Geometry: final body of the model. Coordinates: model frame, mm. A direction names the side the tool comes from. Round coordinates to 2 decimals unless told otherwise and drop trailing zeros. Loops run counter-clockwise (first coordinate to the right, second up) from the corner with the lowest first, then second, coordinate; pieces in that order, holes last. Notation, with made-up numbers: (22, 35) -> (65, 35) arc R32 ccw to (65, 67) -> close; hole circle Ø3 at (43, -6). An arc over 180 degrees is marked (long way). Answer in a Markdown table with one row per item.
```python
from build123d import *

# Parameters (mm, degrees)
AXIAL_START       = 9.7
SKETCH2_R         = 1.65
AXIAL_HOLES_DEPTH = 4


with BuildPart() as part:
    # Axial profile (mm) → Full revolution (revolve)
    with BuildSketch(Plane.XY, mode=Mode.PRIVATE) as full_revolution_sk:
        Polygon((-126, 52), (9.7, 52), (9.7, 32), (13.7, 32), (13.7, 55), (-126, 55), align=None)
    revolve(full_revolution_sk.sketch.rotate(Axis((-110, 0, 0), (1, 0, 0)), 90), axis=Axis((-110, 0, 0), (1, 0, 0)))

    # Sketch2 → Axial holes (cut)
    with BuildSketch(Plane(origin=(0, 0, 0), x_dir=(0, 0, -1), z_dir=(1, 0, 0)).offset(AXIAL_START)):
        with Locations((-34.648232278, 34.648232278)):
            Circle(SKETCH2_R)
        with Locations((-34.648232278, -34.648232278)):
            Circle(SKETCH2_R)
        with Locations((34.648232278, -34.648232278)):
            Circle(SKETCH2_R)
        with Locations((34.648232278, 34.648232278)):
            Circle(SKETCH2_R)
    extrude(amount=AXIAL_HOLES_DEPTH, mode=Mode.SUBTRACT)


solid = part.part
```
Item 1: Section query C-C, the plane x = -15.5. Output: boundary loops of the cut face in (y, z).
Ans:
| item | result |
|---|---|
| outline | circle Ø110 at (0, 0); hole circle Ø104 at (0, 0) |
Item 2: Section query A-A, the plane y = 0. Output: boundary loops of the cut face in (x, z).
Ans:
| item | result |
|---|---|
| outline | (-126, -55) -> (13.7, -55) -> (13.7, -32) -> (9.7, -32) -> (9.7, -52) -> (-126, -52) -> close; (-126, 52) -> (9.7, 52) -> (9.7, 32) -> (13.7, 32) -> (13.7, 55) -> (-126, 55) -> close |
Item 3: Mould query, pull axis Y, two halves, no side actions, for faces 1 (the cylindrical face through (-57.128, 48.794, 25.379)), 2 (the cylindrical face through (11.672, 34.016, 33.124)), 3 (the flat face through (13.7, 24, -24)). Classes: released by +Y, released by -Y, zero draft, split by the parting line, or undercut.
Ans:
| item | result |
|---|---|
| face 1 | split by the parting line |
| face 2 | undercut |
| face 3 | zero draft |
Item 4: Section query D-D, the plane z = -42.5. Output: boundary loops of the cut face in (x, y), and give its area (3 significant figures).
Ans:
| item | result |
|---|---|
| outline | (-126, -34.91) -> (13.7, -34.91) -> (13.7, 34.91) -> (-126, 34.91) -> (-126, 29.96) -> (9.7, 29.96) -> (9.7, -29.96) -> (-126, -29.96) -> close |
| area | 1,620 mm2 |
Item 5: Set-up query: faces 4 (the cylindrical face through (-57.2, 31.641, -41.265)), 5 (the cylindrical face through (11.672, -35.28, 33.124)). Return all of +Z, -Z, +X, -X, +Y, -Y with unobstructed straight access to the full face (end or side cutting, diameter ignored); none if empty.
Ans:
| item | result |
|---|---|
| face 4 | -X |
| face 5 | +X, -X |
Item 6: First-contact query: P1, Ø1, axis at y = -32.5, z = 10, coming from the -X side; P2, Ø3, axis at x = -13.5, y = -16.5, coming from the +Z side (3 decimals); P3, Ø5, axis at x = -89, z = -43, coming from the -Y side; P4, Ø4, axis at y = 34.65, z = 34.65, coming from the +X side. Flat tips, straight axial feed; report the tip coordinate or a pass-through.
Ans:
| item | result |
|---|---|
| P1 | x = 9.7 |
| P2 | z = 52.915 |
| P3 | y = -37.21 |
| P4 | x = 13.7 |
Item 7: Ray query, L1, parallel to Y at x = -75.5, z = 0; L2, parallel to Y at x = -32, z = -43; L3, parallel to Z at x = -88, y = -21. Return the intervals inside material, ascending.
Ans:
| item | result |
|---|---|
| L1 | -55 to -52, 52 to 55 |
| L2 | -34.29 to -29.24, 29.24 to 34.29 |
| L3 | -50.83 to -47.57, 47.57 to 50.83 |
